Here's how the part is built. I have some questions about the finished solid (model axes, mm). Give positions to 0.01 mm unless a question says otherwise; leave off trailing zeros. Order: outer loops, then holes, each group sorted by start corner. A loop starts at its lowest first (then second) coordinate and runs counter-clockwise, first axis right, second up. Notation, with made-up numbers: M 48.5,41 L 79.5,41 A28 ccw 79.5,76 Z; hole C 50,89.25 d5. An arc over 180 degrees is marked long. One line per item, written item: value. Start each with the question number.
from build123d import *

# Parameters (mm, degrees)
ESQUISSE1_R             = 1
ESQUISSE1_W             = 207
ESQUISSE1_H             = 281.553390594
ESQUISSE1_W_2           = 172
ESQUISSE1_H_2           = 280.534461641
BOSS_EXTRU_1_DEPTH      = 8
ENL_V_MAT_EXTRU_2_DEPTH = 4
ENL_V_MAT_EXTRU_3_DEPTH = 4
ESQUISSE6_R             = 4
ENL_V_MAT_EXTRU_4_DEPTH = 6


with BuildPart() as part:
    # Esquisse1 → Boss.-Extru.1 (new body)
    with BuildSketch(Plane.XY):
        with BuildLine():
            Line((-54.650090097, -45.819197646), (-54.650090097, 358.028972494))
            Line((-54.650090097, 358.028972494), (-54.650090097, 722.896071587))
            Line((-54.650090097, 722.896071587), (45.349909903, 722.896071587))
            Line((45.349909903, 722.896071587), (45.349909903, 717.01739193))
            ThreePointArc((45.349909903, 717.01739193), (45.349909903, 714.896071587), (47.471230246, 714.896071587))
            Line((47.471230246, 714.896071587), (143.228589559, 714.896071587))
            ThreePointArc((143.228589559, 714.896071587), (145.349909903, 714.896071587), (145.349909903, 717.01739193))
            Line((145.349909903, 717.01739193), (145.349909903, 722.896071587))
            Line((145.349909903, 722.896071587), (245.349909903, 722.896071587))
            Line((245.349909903, 722.896071587), (245.349909903, 665.01739193))
            ThreePointArc((245.349909903, 665.01739193), (245.349909903, 662.896071587), (247.471230246, 662.896071587))
            Line((247.471230246, 662.896071587), (253.349909903, 662.896071587))
            Line((253.349909903, 662.896071587), (253.349909903, 607.896071587))
            Line((253.349909903, 607.896071587), (247.471230246, 607.896071587))
            ThreePointArc((247.471230246, 607.896071587), (245.349909903, 607.896071587), (245.349909903, 605.774751243))
            Line((245.349909903, 605.774751243), (245.349909903, 555.01739193))
            ThreePointArc((245.349909903, 555.01739193), (245.349909903, 552.896071587), (247.471230246, 552.896071587))
            Line((247.471230246, 552.896071587), (253.349909903, 552.896071587))
            Line((253.349909903, 552.896071587), (253.349909903, 497.896071587))
            Line((253.349909903, 497.896071587), (247.471230246, 497.896071587))
            ThreePointArc((247.471230246, 497.896071587), (245.349909903, 497.896071587), (245.349909903, 495.774751243))
            Line((245.349909903, 495.774751243), (245.349909903, 445.01739193))
            ThreePointArc((245.349909903, 445.01739193), (245.349909903, 442.896071587), (247.471230246, 442.896071587))
            Line((247.471230246, 442.896071587), (253.349909903, 442.896071587))
            Line((253.349909903, 442.896071587), (253.349909903, 387.896071587))
            Line((253.349909903, 387.896071587), (247.471230246, 387.896071587))
            ThreePointArc((247.471230246, 387.896071587), (245.349909903, 387.896071587), (245.349909903, 385.774751243))
            Line((245.349909903, 385.774751243), (245.349909903, 331.302122698))
            ThreePointArc((245.349909903, 331.302122698), (245.349909903, 329.180802354), (247.471230246, 329.180802354))
            Line((247.471230246, 329.180802354), (253.349909903, 329.180802354))
            Line((253.349909903, 329.180802354), (253.349909903, 274.180802354))
            Line((253.349909903, 274.180802354), (247.471230246, 274.180802354))
            ThreePointArc((247.471230246, 274.180802354), (245.349909903, 274.180802354), (245.349909903, 272.059482011))
            Line((245.349909903, 272.059482011), (245.349909903, 221.302122698))
            ThreePointArc((245.349909903, 221.302122698), (245.349909903, 219.180802354), (247.471230246, 219.180802354))
            Line((247.471230246, 219.180802354), (253.349909903, 219.180802354))
            Line((253.349909903, 219.180802354), (253.349909903, 164.180802354))
            Line((253.349909903, 164.180802354), (247.471230246, 164.180802354))
            ThreePointArc((247.471230246, 164.180802354), (245.349909903, 164.180802354), (245.349909903, 162.059482011))
            Line((245.349909903, 162.059482011), (245.349909903, 111.302122698))
            ThreePointArc((245.349909903, 111.302122698), (245.349909903, 109.180802354), (247.471230246, 109.180802354))
            Line((247.471230246, 109.180802354), (253.349909903, 109.180802354))
            Line((253.349909903, 109.180802354), (253.349909903, 54.180802354))
            Line((253.349909903, 54.180802354), (247.471230246, 54.180802354))
            ThreePointArc((247.471230246, 54.180802354), (245.349909903, 54.180802354), (245.349909903, 52.059482011))
            Line((245.349909903, 52.059482011), (245.349909903, -45.819197646))
            Line((245.349909903, -45.819197646), (-54.650090097, -45.819197646))
        make_face()
        with Locations((195.349909903, 718.896071587)):
            Circle(ESQUISSE1_R, mode=Mode.SUBTRACT)
        with Locations(Location((-4.650090097, 718.896071587, 0), (0, 0, 180))):
            Circle(ESQUISSE1_R, mode=Mode.SUBTRACT)
        with Locations((121.849909903, 522.11937629)):
            Rectangle(ESQUISSE1_W, ESQUISSE1_H, mode=Mode.SUBTRACT)
        with Locations((139.349909903, 194.448033175)):
            Rectangle(ESQUISSE1_W_2, ESQUISSE1_H_2, mode=Mode.SUBTRACT)
    extrude(amount=BOSS_EXTRU_1_DEPTH)

    # Esquisse3 → Enlèv. mat.-Extru.2 (cut)
    with BuildSketch(Plane(origin=(0, 0, 0), x_dir=(-1, 0, 0), z_dir=(0, 0, -1))):
        with BuildLine():
            Line((-228.228589559, 339.715263995), (-50.471230246, 339.715263995))
            ThreePointArc((-50.471230246, 339.715263995), (-48.349909903, 339.715263995), (-48.349909903, 337.593943652))
            Line((-48.349909903, 337.593943652), (-48.349909903, 51.302122698))
            ThreePointArc((-48.349909903, 51.302122698), (-48.349909903, 49.180802354), (-50.471230246, 49.180802354))
            Line((-50.471230246, 49.180802354), (-228.228589559, 49.180802354))
            ThreePointArc((-228.228589559, 49.180802354), (-230.349909903, 49.180802354), (-230.349909903, 51.302122698))
            Line((-230.349909903, 51.302122698), (-230.349909903, 337.593943652))
            ThreePointArc((-230.349909903, 337.593943652), (-230.349909903, 339.715263995), (-228.228589559, 339.715263995))
        make_face()
    extrude(amount=-ENL_V_MAT_EXTRU_2_DEPTH, mode=Mode.SUBTRACT)

    # Esquisse5 → Enlèv. mat.-Extru.3 (cut)
    with BuildSketch(Plane(origin=(0, 0, 0), x_dir=(-1, 0, 0), z_dir=(0, 0, -1))):
        with BuildLine():
            Line((-35.349909903, -45.819197646), (-43.849909903, -45.819197646))
            Line((-43.849909903, -45.819197646), (-43.849909903, 712.532944954))
            ThreePointArc((-43.849909903, 712.532944954), (-44.060076233, 714.785905254), (-41.807115933, 714.996071584))
            Line((-41.807115933, 714.996071584), (-37.392703873, 714.996071584))
            ThreePointArc((-37.392703873, 714.996071584), (-35.139743573, 714.785905254), (-35.349909903, 712.532944954))
            Line((-35.349909903, 712.532944954), (-35.349909903, -45.819197646))
        make_face()
    extrude(amount=-ENL_V_MAT_EXTRU_3_DEPTH, mode=Mode.SUBTRACT)

    # Esquisse6 → Enlèv. mat.-Extru.4 (cut)
    with BuildSketch(Plane(origin=(0, 0, 0), x_dir=(-1, 0, 0), z_dir=(0, 0, -1))):
        with Locations((34.650090097, -25.819197646)):
            Circle(ESQUISSE6_R)
    extrude(amount=-ENL_V_MAT_EXTRU_4_DEPTH, mode=Mode.SUBTRACT)


solid = part.part
Item 1: I want a section at D-D on x = 157.5. Write out the boundary of the cut face in (y, z).
Item 2: We'd pull the mould along Y, two halves only. Please class faces 1 (the face through (67, 344, 8)), 2 (the face through (227, 238, 4)): +Y half, -Y half, draft (parallel to the pull), parting line (faces both ways), or undercut.
Item 3: I want a section at B-B on x = 77.5. Write out the boundary of the cut face in (y, z), plus the area to 3 significant figures.
Item 4: I want a section at C-C on y = 653. Write out the boundary of the cut face in (x, z), plus the area to 3 significant figures.
Item 5: Will these pins go through, and if not, where does the flat tip stop? P1, Ø4.5, axis at x = 249, z = 2, coming from the +Y side; P2, Ø1.2, axis at y = 246.5, z = 2.5, coming from the +X side; P3, Ø3, axis at x = 251, z = 2, coming from the -Y side; P4, Ø6, axis at x = 116.5, y = 57.5, coming from the -Z side.
Item 6: I want a section at A-A on y = 126. Write out the boundary of the cut face in (x, z), plus the area to 3 significant figures.
Item 7: Please list where these lines run through material, in increasing order: probe 1 along Y at (x, z) = (223.5, 1.25); probe 2 along X at (y, z) = (276, 0.75); probe 3 along X at (y, z) = (247, 1). Write a range as [from, to].
Answer below:
1. outline: M -45.82,0 L 49.18,0 L 49.18,4 L 54.18,4 L 54.18,8 L -45.82,8 Z; M 334.72,4 L 339.72,4 L 339.72,0 L 381.34,0 L 381.34,8 L 334.72,8 Z; M 662.9,0 L 722.9,0 L 722.9,8 L 662.9,8 Z
2. face 1: draft
2. face 2: undercut
3. outline: M -45.82,0 L 49.18,0 L 49.18,4 L 54.18,4 L 54.18,8 L -45.82,8 Z; M 334.72,4 L 339.72,4 L 339.72,0 L 381.34,0 L 381.34,8 L 334.72,8 Z; M 662.9,0 L 714.9,0 L 714.9,8 L 662.9,8 Z
3. area: 1,550 mm²
4. outline: M -54.65,0 L 18.35,0 L 18.35,8 L -54.65,8 Z; M 225.35,0 L 253.35,0 L 253.35,8 L 225.35,8 Z
4. area: 808 mm²
5. P1: stops at y = 662.9
5. P2: stops at x = 245.35
5. P3: stops at y = 54.18
5. P4: passes through
6. outline: M -54.65,0 L 35.35,0 L 35.35,4 L 43.85,4 L 43.85,0 L 48.35,0 L 48.35,4 L 53.35,4 L 53.35,8 L -54.65,8 Z; M 225.35,4 L 230.35,4 L 230.35,0 L 245.35,0 L 245.35,8 L 225.35,8 Z
6. area: 950 mm²
7. probe 1: y = [-45.82, 49.18], [339.72, 381.34], [662.9, 722.9]
7. probe 2: x = [-54.65, 35.35], [43.85, 48.35], [230.35, 253.35]
7. probe 3: x = [-54.65, 35.35], [43.85, 48.35], [230.35, 245.35]
